Source: CAD feature listing. Evaluate the final solid. Frame: model axes, mm. Give positions to 0.01 mm unless a question says otherwise; leave off trailing zeros. Loops run counter-clockwise (first coordinate to the right, second up) from the corner with the lowest first, then second, coordinate; pieces in that order, holes last. Notation, with made-up numbers: (-3.5, 13.25) - (27.5, 13.25) arc R23 cw to (27.5, 44.25) - close; hole circle Ø5 at (21, 63). An arc over 180 degrees is marked (long way). Put each result on its own line as item: value.
```python
from build123d import *

# Parameters (mm, degrees)
F1_DEPTH = 100
F3_D     = 11


with BuildPart() as f1:
    # F0 (on Top) → F1 (new body)
    with BuildSketch(Plane.XY):
        with BuildLine():
            Line((45, -298.3239697419), (45, -151.9868415357))
            ThreePointArc((45, -151.9868415357), (45.9495370635, -149.0553316858), (48.4375, -147.2372527377))
            ThreePointArc((48.4375, -147.2372527377), (155, 0), (48.4375, 147.2372527377))
            Line((48.4375, 147.2372527377), (40, 144.568322948))
            ThreePointArc((40, 144.568322948), (149.8888164954, 1.8456395549), (43.5443348323, -143.5371914998))
            ThreePointArc((43.5443348323, -143.5371914998), (40.9826422963, -145.343888573), (40, -148.3206043943))
            Line((40, -148.3206043943), (40, -298.3239697419))
            Line((40, -298.3239697419), (45, -298.3239697419))
        make_face()
    extrude(amount=F1_DEPTH)

    # F3 (through all)
    with Locations(Plane.XZ.offset(298.3239697419)):
        with Locations((100, 89), (100, 11)):
            Hole(F3_D / 2)


solid = f1.part
```
1) Material intervals for line 1 along Z through (x, y) = (100, -113.5); line 2 along X through (y, z) = (-161, 74); line 3 along Y through (x, z) = (81.5, 59), sorted ascending. Write a range as [from, to].
Check result:
line 1: [0, 5.5], [16.5, 83.5], [94.5, 100]
line 2: [40, 45]
line 3: [-131.84, -125.88], [125.88, 131.84]
2) Mould query, pull axis X, two halves, no side actions, for faces 1 (the cylindrical face through (101.19, -114.59, 83.63)), 2 (the cylindrical face through (149.83, 4.55, 49.3)), 3 (the flat face through (45, -226, 49)). Classes: pulls with the +X half, pulls with the -X half, needs draft (parallel to the pull), parting line crosses it, or undercut.
Check result:
face 1: undercut
face 2: pulls with the -X half
face 3: pulls with the +X half
3) Section query A-A, the plane z = 11. Output: boundary loops of the cut face in (x, y).
Check result:
outline: (40, -298.32) - (45, -298.32) - (45, -151.99) arc R5 cw to (48.44, -147.24) arc R155 ccw to (94.5, -122.86) - (94.5, -116.43) arc R150.04 cw to (43.54, -143.54) arc R5 ccw to (40, -148.32) - close; (40, 144.57) arc R150.04 cw to (94.5, 116.43) - (94.5, 122.86) arc R155 ccw to (48.44, 147.24) - close; (105.5, -113.56) arc R155 ccw to (105.5, 113.56) - (105.5, 106.55) arc R150.04 cw to (105.5, -106.55) - close
4) Section query C-C, the plane x = 59. Output: boundary loops of the cut face in (y, z), plus the area to 3 significant figures.
Check result:
outline: (-143.33, 0) - (-137.89, 0) - (-137.89, 100) - (-143.33, 100) - close; (137.89, 0) - (143.33, 0) - (143.33, 100) - (137.89, 100) - close
area: 1,090 mm²
5) Pin query (flat end, axial travel): P1, Ø17.5, axis at x = 100, z = 11, coming from the +Y side; P2, Ø12.5, axis at x = 100, z = 11, coming from the +Y side; P3, Ø12.5, axis at x = 100, z = 89, coming from the -Y side; P4, Ø6, axis at x = 59, y = -149, coming from the +Z side. Return the tip coordinate at first contact, or that it passes through.
Check result:
P1: y = 125.29
P2: y = 123.43
P3: y = -123.43
P4: through
6) Section query D-D, the plane z = 42.5. Output: boundary loops of the cut face in (x, y), plus the area to 3 significant figures.
Check result:
outline: (40, -298.32) - (45, -298.32) - (45, -151.99) arc R5 cw to (48.44, -147.24) arc R155 ccw to (48.44, 147.24) - (40, 144.57) arc R150.04 cw to (43.54, -143.54) arc R5 ccw to (40, -148.32) - close
area: 2,740 mm²
7) Section query B-B, the plane x = 100. Output: boundary loops of the cut face in (y, z), plus the area to 3 significant figures.
Check result:
outline: (-118.43, 0) - (-111.73, 0) - (-111.73, 5.5) - (-118.43, 5.5) - close; (-118.43, 16.5) - (-111.73, 16.5) - (-111.73, 83.5) - (-118.43, 83.5) - close; (-118.43, 94.5) - (-111.73, 94.5) - (-111.73, 100) - (-118.43, 100) - close; (111.73, 0) - (118.43, 0) - (118.43, 5.5) - (111.73, 5.5) - close; (111.73, 16.5) - (118.43, 16.5) - (118.43, 83.5) - (111.73, 83.5) - close; (111.73, 94.5) - (118.43, 94.5) - (118.43, 100) - (111.73, 100) - close
area: 1,040 mm²
